from build123d import *

# Parameters (mm, degrees)
SKETCH2_R          = 1.5
CUT_EXTRUDE1_DEPTH = 31
SKETCH3_R          = 3.5
SKETCH3_R_2        = 1.5
CUT_EXTRUDE2_DEPTH = 1


with BuildPart() as part:
    # Sketch1 → Revolve5 (revolve)
    with BuildSketch(Plane.XY):
        with BuildLine():
            Line((-15.473870067, 0), (14.526129933, 0))
            Line((14.526129933, 0), (14.526129933, 2.977982181))
            ThreePointArc((14.526129933, 2.977982181), (14.061170532, 4.260031462), (12.882479574, 4.945979877))
            add(Edge.make_bspline(
                [(12.882479574, 4.945979877), (-0.755720694, 7.415478586), (-13.871264836, 4.756435317)],
                knots=[0.969017626, 0.969017626, 0.969017626, 2.226302938, 2.226302938, 2.226302938], degree=2, weights=[1, 0.808826436, 1]))
            ThreePointArc((-13.871264836, 4.756435317), (-15.022222343, 4.062253989), (-15.473870067, 2.796313536))
            Line((-15.473870067, 2.796313536), (-15.473870067, 0))
        make_face()
    revolve(axis=Axis((-15.473870067, 0, 0), (1, 0, 0)))

    # Sketch2 → Cut-Extrude1 (cut, through all)
    with BuildSketch(Plane(origin=(14.526129933, 0, 0), x_dir=(0, 0, -1), z_dir=(1, 0, 0))):
        Circle(SKETCH2_R)
    extrude(amount=-CUT_EXTRUDE1_DEPTH, mode=Mode.SUBTRACT)

    # Sketch3 → Cut-Extrude2 (cut)
    with BuildSketch(Plane(origin=(14.526129933, 0, 0), x_dir=(0, 0, -1), z_dir=(1, 0, 0))):
        Circle(SKETCH3_R)
        Circle(SKETCH3_R_2, mode=Mode.SUBTRACT)
    cut_extrude2 = extrude(amount=-CUT_EXTRUDE2_DEPTH, mode=Mode.SUBTRACT)

    # Mirror1: Cut-Extrude2 across plane
    add(cut_extrude2.mirror(Plane(origin=(-0.473870067, 0, 0), x_dir=(0, 0, 1), z_dir=(1, 0, 0))), mode=Mode.SUBTRACT)


solid = part.part
Geometry: final body of the model. Coordinates: model frame, mm. A direction names the side the tool comes from. Coordinates: 2 decimals unless noted, no trailing zeros.
(1) First-contact query: pin 1 (2 mm diameter, centred on y = -1.5, z = 1, fed in from +X); pin 2 (6.5 mm diameter, centred on y = 0, z = 0, fed in from -X); pin 3 (1.8 mm diameter, centred on y = 0, z = 0, fed in from -X); pin 4 (1.5 mm diameter, centred on x = 1.5, z = -2, fed in from -Y). Flat tips, straight axial feed; report the tip coordinate or a pass-through.
(2) Material intervals for probe 1 along Y at (x, z) = (-8.75, 0.25); probe 2 along Y at (x, z) = (14, 0); probe 3 along Z at (x, y) = (9, 0.75), sorted ascending.
(3) Access query for faces 1 (the face through (-14.916, -1.341, -3.233)), 2 (the face through (13.998, -1.341, -3.233)), 3 (the face through (-0.28, 0.07, 1.5)). Directions: +Z, -Z, +X, -X, +Y, -Y. A direction counts if a zero-diameter tool reaches every point of the face in a straight line with its end or side. Return the directions, or none.
(4) Draft query along Z for faces 4 (the face through (13.526, -2, 0)), 5 (the face through (-14.474, -2, 0)). Return one class per face: pulls with the +Z half, pulls with the -Z half, needs draft (parallel to the pull), parting line crosses it, or undercut.
Solution:
1. pin 1: stops at x = 13.53
1. pin 2: stops at x = -14.47
1. pin 3: passes through
1. pin 4: stops at y = -5.86
2. probe 1: y = -5.53 to -1.48, 1.48 to 5.53
2. probe 2: y = -4.33 to -3.5, 3.5 to 4.33
2. probe 3: z = -5.46 to -1.3, 1.3 to 5.46
3. face 1: -X
3. face 2: +X
3. face 3: +X, -X
4. face 4: undercut
4. face 5: undercut
